Input: part model. Units: mm. Frame: model coordinates. Face numbers are marked on the shaded views. A direction names the side the tool comes from. Coordinates: 2 decimals unless noted, no trailing zeros. Write each loop counter-clockwise with the first axis right and the second up, starting at its lowest first coordinate (ties: lowest second). Pieces come first, ordered by that corner, then holes. Notation, with made-up numbers: (51, -33) -> (84, -33) arc R17 ccw to (84, -14) -> close; hole circle Ø8 at (-26.5, 69.25). An arc over 180 degrees is marked (long way). Use one line per item in the form item = value. Start each with the question number.
(1) Cut plane A-A on z = 5.75. Return the cut outline in (x, y).
(2) Cut plane B-B on x = 8. Return the cut outline in (y, z).
(3) Ray query, line 1 along Y through (x, z) = (5.5, 6.25); line 2 along Y through (x, z) = (-1.5, 3); line 3 along X through (y, z) = (-1.25, 10). Return the intervals inside material, ascending.
(4) Set-up query: the marked faces 5, 6 and 7. Return all of +Z, -Z, +X, -X, +Y, -Y with unobstructed straight access to the full face (end or side cutting, diameter ignored); none if empty.
(5) Cut plane C-C on z = 10.75. Return the cut outline in (x, y) (3 decimals).
(6) Pull-direction query (X, two-part tool) for the marked faces 1, 2, 3 and 4; classes: released by +X, released by -X, zero draft, split by the parting line, or undercut.
(7) Cut plane D-D on y = -2. Return the cut outline in (x, z).
```python
from build123d import *

# Parameters (mm, degrees)
F0_W     = 31.8516
F0_H     = 7.8486
F1_DEPTH = 9.6774
F2_R     = 2.4638
F3_DEPTH = 1.8034
F5_W     = 28.7528
F5_H     = 4.7498
F5_R     = 1.5494
F6_DEPTH = 8.0772


with BuildPart() as f1:
    # F0 (on Top) → F1 (new body)
    with BuildSketch(Plane.XY):
        Rectangle(F0_W, F0_H)
    extrude(amount=F1_DEPTH)

    # F2 (on face) → F3 (join)
    with BuildSketch(Plane.XY.offset(9.6774)):
        with Locations((-4.064, 0)):
            Circle(F2_R)
        with Locations((3.937, 0)):
            Circle(F2_R)
        with Locations((11.938, 0)):
            Circle(F2_R)
        with Locations((-12.065, 0)):
            Circle(F2_R)
    extrude(amount=F3_DEPTH)

    # F5 (on face) → F6 (cut)
    with BuildSketch(Plane(origin=(0, 0, 0), x_dir=(1, 0, 0), z_dir=(0, 0, -1))):
        Rectangle(F5_W, F5_H)
        with Locations((-8.1407, 0)):
            Circle(F5_R, mode=Mode.SUBTRACT)
        with Locations((-0.1651, 0)):
            Circle(F5_R, mode=Mode.SUBTRACT)
        with Locations((7.8105, 0)):
            Circle(F5_R, mode=Mode.SUBTRACT)
    extrude(amount=-F6_DEPTH, mode=Mode.SUBTRACT)


solid = f1.part
```
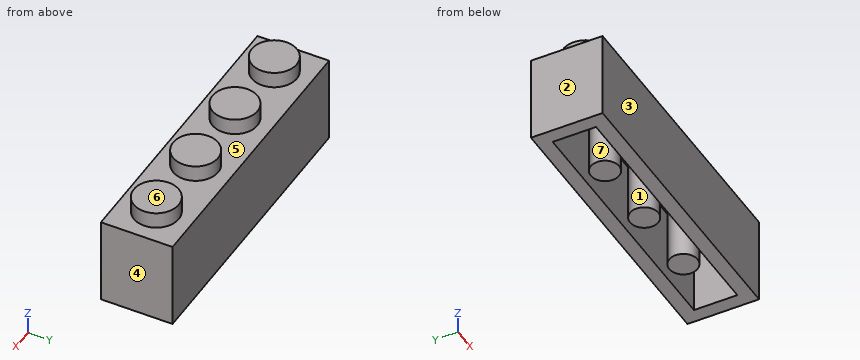
Values:
q1.outline = (-15.93, -3.92) -> (15.93, -3.92) -> (15.93, 3.92) -> (-15.93, 3.92) -> close; circle Ø3.1 at (-8.14, 0); circle Ø3.1 at (-0.17, 0); circle Ø3.1 at (7.81, 0); hole (-14.38, -2.37) -> (14.38, -2.37) -> (14.38, 2.37) -> (-14.38, 2.37) -> close
q2.outline = (-3.92, 0) -> (-2.37, 0) -> (-2.37, 8.08) -> (-1.54, 8.08) -> (-1.54, 0) -> (1.54, 0) -> (1.54, 8.08) -> (2.37, 8.08) -> (2.37, 0) -> (3.92, 0) -> (3.92, 9.68) -> (-3.92, 9.68) -> close
q3.line_1 = -3.92 to -2.37, 2.37 to 3.92
q3.line_2 = -3.92 to -2.37, -0.79 to 0.79, 2.37 to 3.92
q3.line_3 = -14.19 to -9.94, -6.19 to -1.94, 1.81 to 6.06, 9.81 to 14.06
q4.face_5 = +Z
q4.face_6 = +Z, +X, -X, +Y, -Y
q4.face_7 = -Z
q5.outline = circle Ø4.928 at (-12.065, 0); circle Ø4.928 at (-4.064, 0); circle Ø4.928 at (3.937, 0); circle Ø4.928 at (11.938, 0)
q6.face_1 = undercut
q6.face_2 = released by -X
q6.face_3 = zero draft
q6.face_4 = released by +X
q7.outline = (-15.93, 0) -> (-14.38, 0) -> (-14.38, 8.08) -> (14.38, 8.08) -> (14.38, 0) -> (15.93, 0) -> (15.93, 9.68) -> (13.38, 9.68) -> (13.38, 11.48) -> (10.5, 11.48) -> (10.5, 9.68) -> (5.38, 9.68) -> (5.38, 11.48) -> (2.5, 11.48) -> (2.5, 9.68) -> (-2.63, 9.68) -> (-2.63, 11.48) -> (-5.5, 11.48) -> (-5.5, 9.68) -> (-10.63, 9.68) -> (-10.63, 11.48) -> (-13.5, 11.48) -> (-13.5, 9.68) -> (-15.93, 9.68) -> close
